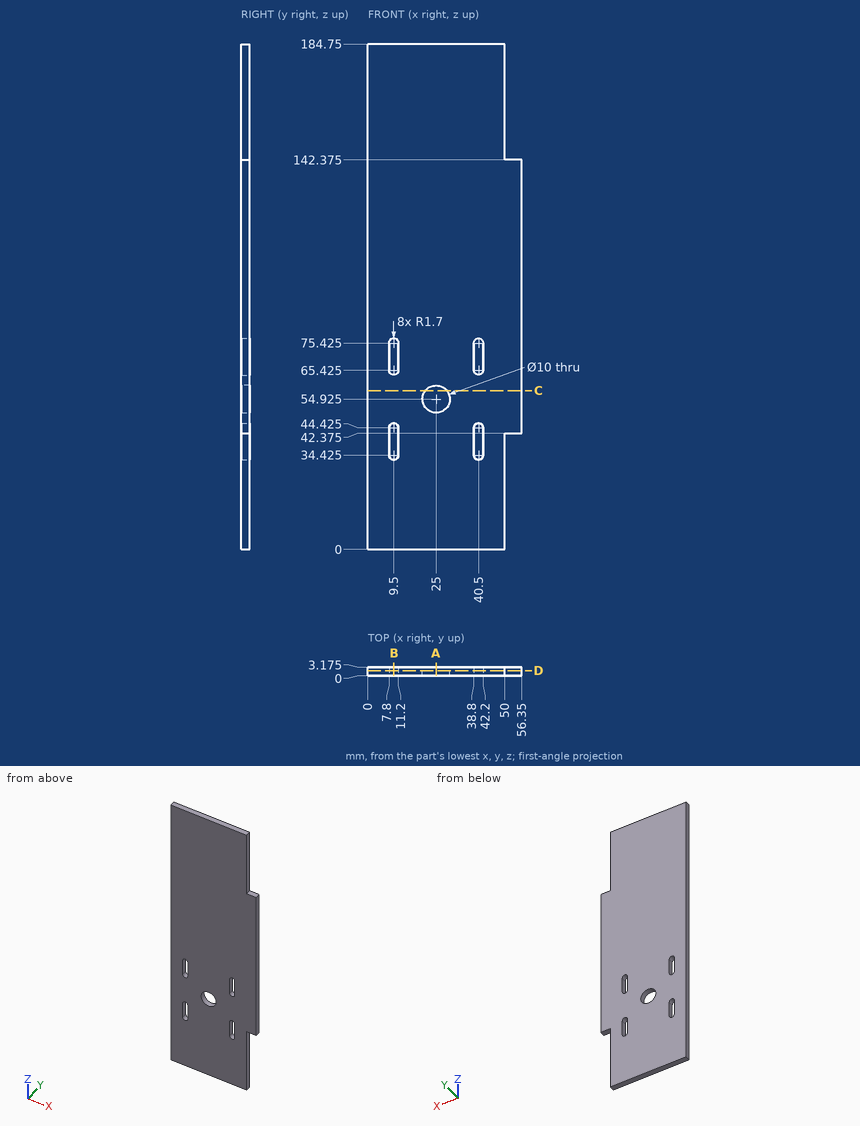
Geometry: see drawing. Coordinates: mm, zero at the bounding-box minimum. Give positions to 0.01 mm unless a question says otherwise; leave off trailing zeros. Order: outer loops, then holes, each group sorted by start corner. A loop starts at its lowest first (then second) coordinate and runs counter-clockwise, first axis right, second up. Notation, with made-up numbers: M 56,2 L 77,2 A28 ccw 77,36 Z; hole C 22,-3 d7. An arc over 180 degrees is marked long. Answer as CSV lines item,"result". Start each with the question number.
1) Cut plane D-D (y = 2). Output: boundary loops of the cut face in (x, z) (3 decimals), then the cut area to 3 significant figures.
2) First-contact query: P1, Ø1.6, axis at y = 1.5, z = 69, coming from the -X side; P2, Ø1.6, axis at y = 2, z = 41, coming from the +X side; P3, Ø6, axis at x = 25, z = 54.925, coming from the +Y side. Flat tips, straight axial feed; report the tip coordinate or a pass-through.
3) Line query: line 1 (Z direction, x = 39.5, y = 1.5); line 2 (X direction, y = 2.55, z = 28); line 3 (X direction, y = 0.25, z = 52). Output: solid intervals per line, ascending. Write a range as from..to.
4) Cut plane A-A (x = 25). Output: boundary loops of the cut face in (y, z) (3 decimals).
5) Cut plane C-C (z = 58). Output: boundary loops of the cut face in (x, y) (3 decimals), then the cut area to 3 significant figures.
6) Cut plane B-B (x = 9.5). Output: boundary loops of the cut face in (y, z) (3 decimals).
Findings below:
1,outline,"M 0,0 L 50,0 L 50,42.375 L 56.35,42.375 L 56.35,142.375 L 50,142.375 L 50,184.75 L 0,184.75 Z; hole M 7.8,34.425 A1.7 ccw 11.2,34.425 L 11.2,44.425 A1.7 ccw 7.8,44.425 Z; hole M 7.8,65.425 A1.7 ccw 11.2,65.425 L 11.2,75.425 A1.7 ccw 7.8,75.425 Z; hole C 25,54.925 d10; hole M 38.8,34.425 A1.7 ccw 42.2,34.425 L 42.2,44.425 A1.7 ccw 38.8,44.425 Z; hole M 38.8,65.425 A1.7 ccw 42.2,65.425 L 42.2,75.425 A1.7 ccw 38.8,75.425 Z"
1,area,"9,620 mm²"
2,P1,"stops at x = 0"
2,P2,"stops at x = 50"
2,P3,"passes through"
3,line 1,"z = 0..33.05, 45.8..64.05, 76.8..184.75"
3,line 2,"x = 0..50"
3,line 3,"x = 0..20.94, 29.06..56.35"
4,outline,"M 0,0 L 3.175,0 L 3.175,49.925 L 0,49.925 Z; M 0,59.925 L 3.175,59.925 L 3.175,184.75 L 0,184.75 Z"
5,outline,"M 0,0 L 21.057,0 L 21.057,3.175 L 0,3.175 Z; M 28.943,0 L 56.35,0 L 56.35,3.175 L 28.943,3.175 Z"
5,area,"154 mm²"
6,outline,"M 0,0 L 3.175,0 L 3.175,32.725 L 0,32.725 Z; M 0,46.125 L 3.175,46.125 L 3.175,63.725 L 0,63.725 Z; M 0,77.125 L 3.175,77.125 L 3.175,184.75 L 0,184.75 Z"
